from build123d import *

# Parameters (mm, degrees)
SKETCH_1_W                = 100
SKETCH_1_H                = 1060
EXTRUDE_1_DEPTH           = 12
SKETCH_2_R                = 36.6
CUT_EXTRUDE_1_DEPTH       = 533.488497528
HOLE_WIZARD_M5_1_D        = 4.2
HOLE_WIZARD_M6_1_D        = 5
HOLE_WIZARD_1_D           = 6.6
HOLE_WIZARD_1_CBORE_D     = 11
HOLE_WIZARD_1_CBORE_DEPTH = 6.8
HOLE_WIZARD_M3_1_D        = 2.5
HOLE_WIZARD_M3_1_DEPTH    = 7.5
HOLE_WIZARD_M3_1_TIP      = 0.751075774
HOLE_WIZARD_1_2_D         = 12
HOLE_WIZARD_M6_2_D        = 5
CHAMFER_1_SIZE            = 2


with BuildPart() as part:
    # 草图1 → 凸台-拉伸1 (new body)
    with BuildSketch(Plane(origin=(0, 0, 0), x_dir=(1, 0, 0), z_dir=(0, 1, 0))):
        Rectangle(SKETCH_1_W, SKETCH_1_H)
    extrude(amount=EXTRUDE_1_DEPTH)

    # 草图2 → 切除-拉伸1 (cut, through all)
    with BuildSketch(Plane(origin=(0, 12, 0), x_dir=(1, 0, 0), z_dir=(0, 1, 0))):
        with Locations(Location((0, 475, 0), (0, 0, 270))):
            Circle(SKETCH_2_R)
        with BuildLine():
            Line((5, -443.5), (5, -458.5))
            ThreePointArc((5, -458.5), (0, -463.5), (-5, -458.5))
            Line((-5, -458.5), (-5, -443.5))
            ThreePointArc((-5, -443.5), (0, -438.5), (5, -443.5))
        make_face()
    extrude(amount=-CUT_EXTRUDE_1_DEPTH, mode=Mode.SUBTRACT)

    # M5 螺纹孔1 (through all)
    with Locations(Plane(origin=(0, 12, 0), x_dir=(1, 0, 0), z_dir=(0, 1, 0))):
        with Locations((-34.7, 509.7), (34.7, 509.7), (34.7, 440.3), (-34.7, 440.3)):
            Hole(HOLE_WIZARD_M5_1_D / 2)

    # M6 螺纹孔1 (through all)
    with Locations(Plane(origin=(0, 12, 0), x_dir=(1, 0, 0), z_dir=(0, 1, 0))):
        with Locations((-40, 327.5), (-40, 282.5), (40, 282.5), (40, 327.5)):
            Hole(HOLE_WIZARD_M6_1_D / 2)

    # Hole Wizard 1 (through all)
    with Locations(Plane(origin=(0, 12, 0), x_dir=(1, 0, 0), z_dir=(0, 1, 0))):
        with Locations((-44, -448), (-44, -478), (44, -478), (44, -448)):
            CounterBoreHole(HOLE_WIZARD_1_D / 2, HOLE_WIZARD_1_CBORE_D / 2, HOLE_WIZARD_1_CBORE_DEPTH)

    # M3 螺纹孔1
    with Locations(Plane(origin=(0, 12, 0), x_dir=(1, 0, 0), z_dir=(0, 1, 0))):
        with Locations((-4, -381), (-4, -321), (-4, 427), (4, 427), (4, -321), (4, -381)):
            Hole(HOLE_WIZARD_M3_1_D / 2, depth=HOLE_WIZARD_M3_1_DEPTH)
            with Locations((0, 0, -(HOLE_WIZARD_M3_1_DEPTH + HOLE_WIZARD_M3_1_TIP / 2))):  # 118° drill point
                Cone(0, HOLE_WIZARD_M3_1_D / 2, HOLE_WIZARD_M3_1_TIP, mode=Mode.SUBTRACT)

    # Hole Wizard 1 2 (through all)
    with Locations(Plane(origin=(0, 12, 0), x_dir=(1, 0, 0), z_dir=(0, 1, 0))):
        with Locations((0, 385), (0, -279), (0, -423)):
            Hole(HOLE_WIZARD_1_2_D / 2)

    # M6 螺纹孔2 (through all)
    with Locations(Plane(origin=(0, 12, 0), x_dir=(1, 0, 0), z_dir=(0, 1, 0))):
        with Locations((-40, 520), (40, 520), (40, -520), (-40, -520), (0, 365), (0, 0), (0, -259)):
            Hole(HOLE_WIZARD_M6_2_D / 2)

    # 倒角1
    chamfer_1_edges = [part.edges().sort_by_distance(p)[0] for p in [
        (50, 6, 530),
        (-50, 6, 530),
    ]]
    chamfer(chamfer_1_edges, length=CHAMFER_1_SIZE)


solid = part.part
Verification items for the finished model (mm, model axes). Give positions to 0.01 mm unless a question says otherwise; leave off trailing zeros. Write each loop counter-clockwise with the first axis right and the second up, starting at its lowest first coordinate (ties: lowest second). Pieces come first, ordered by that corner, then holes. Notation, with made-up numbers: M 86.25,-24.75 L 100.25,-24.75 A26 cw 100.25,2.25 Z; hole C -22.5,-40 d11. An arc over 180 degrees is marked long. Use CSV: the item, a comma, the result in double quotes.
1) Cross-section at C-C (y = 7). State how many separate pieces and enclosed holes the cut face has, plus the area to 3 significant figures.
Final values:
separate pieces,"1"
enclosed holes,"30"
area,"101,000 mm²"
2) Release check for a two-part mould opening along Z. For faces 1 (the face through (-1, 12, -7)), 2 (the face through (10.99, 6.08, -440.09)) record: released by +Z, released by -Z, zero draft, split by the parting line, or undercut.
Final values:
face 1,"zero draft"
face 2,"undercut"
3) Material ranges on line 1 along Z through (x, y) = (-44, 1.3); line 2 along Z through (x, y) = (-43, 1); line 3 along Z through (x, y) = (4, 2.75), recorded low to high.
Final values:
line 1,"-530 to 444.7, 451.3 to 474.7, 481.3 to 530"
line 2,"-530 to 444.86, 451.14 to 474.86, 481.14 to 530"
line 3,"-530 to -511.38, -438.62 to -389.47, -380.53 to 274.53, 283.47 to 418.53, 427.47 to 440.5, 461.5 to 530"
4) Go/stop test with a flat-tipped pin: pin 1 Ø12 at (x, z) = (-21, 344) entering from -Y. Record where the tip stops, or that it passes through.
Final values:
pin 1,"y = 0"
5) Cross-section at B-B (x = 21.5). Enter the section's corners in (y, z).
Final values:
outline,"M 0,-530 L 12,-530 L 12,-504.62 L 0,-504.62 Z; M 0,-445.38 L 12,-445.38 L 12,530 L 0,530 Z"
6) Cross-section at A-A (z = -475). Enter the section's corners in (x, y).
Final values:
outline,"M -50,0 L -36.6,0 L -36.6,12 L -50,12 Z; M 36.6,0 L 50,0 L 50,12 L 36.6,12 Z"
